```python
from build123d import *

# Parameters (mm, degrees)
F0_W      = 25.4
F0_H      = 50.8
F0_H_2    = 25.4
F0_W_2    = 152.4
F1_DEPTH  = 101.6
F2_W      = 50.8
F2_H      = 50.8
F3_DEPTH  = 304.8
F4_W      = 50.8
F4_H      = 50.8
F5_DEPTH  = 2489.2
F6_W      = 50.8
F6_H      = 50.8
F7_DEPTH  = 254
F8_W      = 152.4867629528
F8_H      = 25.4
F9_DEPTH  = 101.6
F11_D     = 25.4
F11_DEPTH = 2540
F11_TIP   = 7.6309298617


with BuildPart() as f1:
    # F0 (on Top) → F1 (new body)
    with BuildSketch(Plane.XY):
        with Locations((-86.6702721953, 35.7780026045)):
            Rectangle(F0_W, F0_H)
        with Locations((-86.6702721953, -2.3219973955)):
            Rectangle(F0_W, F0_H_2)
        with Locations((2.2297278047, -2.3219973955)):
            Rectangle(F0_W_2, F0_H_2)
        with Locations((-86.6702721953, 73.8780026045)):
            Rectangle(F0_W, F0_H_2)
        with Locations((2.2297278047, 73.8780026045)):
            Rectangle(F0_W_2, F0_H_2)
    extrude(amount=F1_DEPTH)

    # F2 (on face) → F3 (join)
    with BuildSketch(Plane(origin=(0, 86.5780026045, 0), x_dir=(-1, 0, 0), z_dir=(0, 1, 0))):
        with Locations((73.9702721953, 76.2)):
            Rectangle(F2_W, F2_H)
    extrude(amount=F3_DEPTH)

    # F4 (on face) → F5 (join)
    with BuildSketch(Plane.XY.offset(101.6)):
        with Locations((-73.9702721953, 365.9780026045)):
            Rectangle(F4_W, F4_H)
    extrude(amount=F5_DEPTH)

    # F6 (on face) → F7 (join)
    with BuildSketch(Plane.XZ.offset(-340.5780026045)):
        with Locations((-73.9702721953, 2565.4)):
            Rectangle(F6_W, F6_H)
    extrude(amount=F7_DEPTH)

    # F8 (on face) → F9 (join)
    with BuildSketch(Plane(origin=(0, 0, 2540), x_dir=(1, 0, 0), z_dir=(0, 0, -1))):
        Polygon((-99.3702721953, -61.1780026045), (-99.3702721953, -86.5780026045), (78.4297278047, -86.5780026045), (78.4297278047, -61.1780026045), (-73.9702721953, -61.1780026045), align=None)
        Polygon((-99.3702721953, 15.0219973955), (-99.3702721953, -61.1780026045), (-73.9702721953, -61.1780026045), (-73.9702721953, -10.3780026045), (-73.9702721953, 15.0219973955), align=None)
        with Locations((2.2731092811, 2.3219973955)):
            Rectangle(F8_W, F8_H)
    extrude(amount=-F9_DEPTH)

    # F11
    with Locations(Plane.XY.offset(2590.8)):
        with Locations((-73.9702721953, 162.7780026045)):
            Hole(F11_D / 2, depth=F11_DEPTH)
            with Locations((0, 0, -(F11_DEPTH + F11_TIP / 2))):  # 118° drill point
                Cone(0, F11_D / 2, F11_TIP, mode=Mode.SUBTRACT)


solid = f1.part
```
Source: CAD feature listing. Evaluate the final solid. Frame: model axes, mm. A direction names the side the tool comes from. Give positions to 0.01 mm unless a question says otherwise; leave off trailing zeros. Loops run counter-clockwise (first coordinate to the right, second up) from the corner with the lowest first, then second, coordinate; pieces in that order, holes last. Notation, with made-up numbers: (36, -32) - (68, -32) arc R31 cw to (68, -6) - close; hole circle Ø10 at (61.25, 88). An arc over 180 degrees is marked (long way). Use CSV: the item, a comma, the result in double quotes.
1) Set-up query: faces 4 (the flat face through (-48.57, 341, 1127)), 5 (the flat face through (-74, 340.578, 1304)), 6 (the flat face through (8, 86.578, 2590)), 7 (the flat face through (-73.97, 36, 2590)). Return all of +Z, -Z, +X, -X, +Y, -Y with unobstructed straight access to the full face (end or side cutting, diameter ignored); none if empty.
Worked out:
face 4,"+Z, -Z, +X, +Y"
face 5,"+X, -X, -Y"
face 6,"+Z, +X, +Y"
face 7,"+Z, -Z, +X"
2) Cut plane B-B (x = -10). Output: boundary loops of the cut face in (y, z).
Worked out:
outline,"(-15.02, 0) - (10.38, 0) - (10.38, 101.6) - (-15.02, 101.6) - close; (-15.02, 2540) - (10.38, 2540) - (10.38, 2641.6) - (-15.02, 2641.6) - close; (61.18, 0) - (86.58, 0) - (86.58, 101.6) - (61.18, 101.6) - close; (61.18, 2540) - (86.58, 2540) - (86.58, 2641.6) - (61.18, 2641.6) - close"
3) Line query: line 1 (Z direction, x = 27, y = 83); line 2 (Z direction, x = -74.5, y = 266.5); line 3 (Y direction, x = -83.5, z = 1331.5). Output: solid intervals per line, ascending.
Worked out:
line 1,"z = 0 to 101.6, 2540 to 2641.6"
line 2,"z = 50.8 to 101.6, 2540 to 2590.8"
line 3,"y = 340.58 to 391.38"
4) Pin query (flat end, axial travel): P1, Ø4, axis at x = -49, y = 130.5, coming from the +Z side; P2, Ø20.5, axis at y = 73, z = 2565.5, coming from the +X side; P3, Ø4, axis at y = 340.5, z = 773.5, coming from the +X side. Return the tip coordinate at first contact, or that it passes through.
Worked out:
P1,"stops at z = 2590.8"
P2,"stops at x = 78.43"
P3,"stops at x = -48.57"
5) Cut plane C-C (z = 2166). Output: boundary loops of the cut face in (x, y).
Worked out:
outline,"(-99.37, 340.58) - (-48.57, 340.58) - (-48.57, 391.38) - (-99.37, 391.38) - close"
6) Cut plane A-A (y = 281). Output: boundary loops of the cut face in (x, z).
Worked out:
outline,"(-99.37, 50.8) - (-48.57, 50.8) - (-48.57, 101.6) - (-99.37, 101.6) - close; (-99.37, 2540) - (-48.57, 2540) - (-48.57, 2590.8) - (-99.37, 2590.8) - close"
7) Mould query, pull axis Z, two halves, no side actions, for faces 1 (the flat face through (-51, 121, 2540)), 2 (the flat face through (-74, 241, 2590.8)), 3 (the flat face through (1, 10.378, 2590)). Classes: +Z half, -Z half, draft (parallel to the pull), parting line (faces both ways), or undercut.
Worked out:
face 1,"undercut"
face 2,"+Z half"
face 3,"draft"
